```python
from build123d import *

# Parameters (mm, degrees)
F0_R      = 14.5
F1_DEPTH  = 25
F2_R      = 14.5
F3_DEPTH  = 3
F4_R      = 2.5
F5_DEPTH  = 25
F0_R_2    = 3
F6_DEPTH  = 30
F8_DEPTH  = 25
F9_DEPTH  = 3.5
F10_DEPTH = 30
F11_R     = 5


# Not quite as in the source:
# - a feature names something its author has since deleted; it is built from what else it names


with BuildPart() as f1:
    # F0 (on Top) → F1 (new body)
    with BuildSketch(Plane.XY):
        with BuildLine():
            Line((-44.2576195002, 24.5322410017), (-44.2576195002, -25.4677589983))
            Line((-44.2576195002, -25.4677589983), (-40.7576195002, -25.4677589983))
            Line((-40.7576195002, -25.4677589983), (-40.7576195002, 34.0321085225))
            Line((-40.7576195002, 34.0321085225), (26.7423804998, 34.0321085225))
            Line((26.7423804998, 34.0321085225), (26.7423804998, 19.5322410017))
            ThreePointArc((26.7423804998, 19.5322410017), (57.445862821, 6.7799260387), (44.8114401571, 37.5321085225))
            Line((44.8114401571, 37.5321085225), (44.6733208426, 37.5321085225))
            Line((44.6733208426, 37.5321085225), (-44.2576195002, 37.5321085225))
            Line((-44.2576195002, 37.5321085225), (-44.2576195002, 24.5322410017))
        make_face()
        with Locations((44.7423804998, 19.5322410017)):
            Circle(F0_R, mode=Mode.SUBTRACT)
    extrude(amount=F1_DEPTH)

    # F2 (on face) → F3 (join)
    with BuildSketch(Plane.XY.offset(25)):
        with BuildLine():
            ThreePointArc((26.7423804998, 19.5322410017), (29.5038185973, 9.9517279079), (36.9408506267, 3.3107696863))
            ThreePointArc((36.9408506267, 3.3107696863), (62.2844095115, 15.4977375434), (44.8114401571, 37.5321085225))
            Line((44.8114401571, 37.5321085225), (-44.2576195002, 37.5321085225))
            Line((-44.2576195002, 37.5321085225), (-44.2576195002, -25.4677589983))
            Line((-44.2576195002, -25.4677589983), (-40.7576195002, -25.4677589983))
            Line((-40.7576195002, -25.4677589983), (-40.7576195002, -15.0916781276))
            Line((-40.7576195002, -15.0916781276), (-40.7576195002, 34.0321085225))
            Line((-40.7576195002, 34.0321085225), (26.7423804998, 34.0321085225))
            Line((26.7423804998, 34.0321085225), (26.7423804998, 19.5322410017))
        make_face()
        with Locations((44.7423804998, 19.5322410017)):
            Circle(F2_R, mode=Mode.SUBTRACT)
    extrude(amount=-F3_DEPTH)

    # F4 (on face) → F5 (cut)
    with BuildSketch(Plane(origin=(-44.2576195002, 0, 0), x_dir=(0, -1, 0), z_dir=(-1, 0, 0))):
        with Locations((12.9677589983, 12.5)):
            Circle(F4_R)
    extrude(amount=-F5_DEPTH, mode=Mode.SUBTRACT)

    # F0 (on Top) → F6 (cut)
    with BuildSketch(Plane.XY):
        with Locations((44.7423804998, 19.5322410017)):
            Circle(F0_R_2)
    extrude(amount=F6_DEPTH, mode=Mode.SUBTRACT)

    # F4 (on face) → F8 (cut)
    with BuildSketch(Plane(origin=(-44.2576195002, 0, 0), x_dir=(0, -1, 0), z_dir=(-1, 0, 0))):
        with Locations((-22.0322410017, 12.5)):
            Circle(F4_R)
    extrude(amount=-F8_DEPTH, mode=Mode.SUBTRACT)

    # F2 (on face) → F9 (join)
    with BuildSketch(Plane.XY.offset(25)):
        with BuildLine():
            Line((18.9116307646, 10.5619383976), (36.9408506267, 3.3107696863))
            ThreePointArc((36.9408506267, 3.3107696863), (29.5038185973, 9.9517279079), (26.7423804998, 19.5322410017))
            Line((26.7423804998, 19.5322410017), (26.7423804998, 34.0321085225))
            Line((26.7423804998, 34.0321085225), (-40.7576195002, 34.0321085225))
            Line((-40.7576195002, 34.0321085225), (-40.7576195002, -15.0916781276))
            Line((-40.7576195002, -15.0916781276), (-14.5708816946, 10.5619383976))
            Line((-14.5708816946, 10.5619383976), (18.9116307646, 10.5619383976))
        make_face()
        with Locations((44.7423804998, 19.5322410017)):
            Circle(F2_R)
    extrude(amount=-F9_DEPTH)

    # F0 (on Top) → F10 (cut)
    with BuildSketch(Plane.XY):
        with Locations((44.7423804998, 19.5322410017)):
            Circle(F0_R_2)
    extrude(amount=F10_DEPTH, mode=Mode.SUBTRACT)

    # F11
    f11_edges = [f1.edges().sort_by_distance(p)[0] for p in [
        (26.74238, 34.032109, 10.75),
        (26.74238, 26.782175, 21.5),
        (-7.00762, 34.032109, 21.5),
        (-40.75762, 34.032109, 10.75),
        (-40.75762, 9.470215, 21.5),
    ]]
    fillet(f11_edges, radius=F11_R)


solid = f1.part
```
Source: CAD feature listing. Evaluate the final solid. Frame: model axes, mm. A direction names the side the tool comes from. Round coordinates to 2 decimals unless told otherwise and drop trailing zeros. Loops run counter-clockwise (first coordinate to the right, second up) from the corner with the lowest first, then second, coordinate; pieces in that order, holes last.
(1) Contact query for flat-ended pins moving along their axis: pin 1 Ø6 at (y, z) = (22.03, 12.5) entering from -X; pin 2 Ø1.5 at (x, z) = (-4.5, 12) entering from -Y; pin 3 Ø23 at (x, y) = (44.74, 19.53) entering from -Z; pin 4 Ø3 at (x, z) = (45, 12.5) entering from -Y. Output: stop coordinate, or through.
From the geometry:
pin 1: stops at x = -44.26
pin 2: stops at y = 34.03
pin 3: stops at z = 21.5
pin 4: stops at y = 1.53
(2) Material intervals for probe 1 along X at (y, z) = (13, 12.5); probe 2 along X at (y, z) = (21.5, 8); probe 3 along Y at (x, z) = (-31, 15.25), sorted ascending.
From the geometry:
probe 1: x = -44.26 to -40.76, 27.97 to 31.8, 57.69 to 61.52
probe 2: x = -44.26 to -40.76, 26.74 to 30.38, 59.11 to 62.63
probe 3: y = 34.03 to 37.53
(3) Section query D-D (y = -12.5). Output: boundary loops of the cut face in (x, z), and give its area (3 significant figures).
From the geometry:
outline: (-44.26, 0) - (-40.76, 0) - (-40.76, 10.04) - (-44.26, 10.04) - close; (-44.26, 14.96) - (-40.76, 14.96) - (-40.76, 16.5) arc R5 cw to (-38.11, 20.91) - (-38.11, 25) - (-44.26, 25) - close
area: 84.5 mm2
(4) Section query A-A (z = 12.5). Output: boundary loops of the cut face in (x, y).
From the geometry:
outline: (-44.26, -25.47) - (-40.76, -25.47) - (-40.76, -15.47) - (-44.26, -15.47) - close; (-44.26, -10.47) - (-40.76, -10.47) - (-40.76, 19.53) - (-44.26, 19.53) - close; (-44.26, 24.53) - (-40.76, 24.53) - (-40.76, 29.03) arc R5 cw to (-35.76, 34.03) - (21.74, 34.03) arc R5 cw to (26.74, 29.03) - (26.74, 19.53) arc R18 ccw (long way) to (44.81, 37.53) - (-44.26, 37.53) - close; hole circle Ø29 at (44.74, 19.53)
(5) Access query for faces 4 (the flat face through (48, 20, 21.5)), 5 (the flat face through (-7, 34.032, 8)), 6 (the flat face through (2, 10.562, 23)), 7 (the cylindrical face through (-42.53, 22.57, 10.06)). Directions: +Z, -Z, +X, -X, +Y, -Y. A direction counts if a zero-diameter tool reaches every point of the face in a straight line with its end or side. Return the directions, or none.
From the geometry:
face 4: -Z
face 5: -Z, -Y
face 6: +Z, -Z, -Y
face 7: -X
(6) Section query C-C (x = -10). Output: boundary loops of the cut face in (y, z).
From the geometry:
outline: (10.56, 21.5) - (29.03, 21.5) arc R5 cw to (34.03, 16.5) - (34.03, 0) - (37.53, 0) - (37.53, 25) - (10.56, 25) - close
(7) Section query B-B (z = 22.75). Output: boundary loops of the cut face in (x, y).
From the geometry:
outline: (-44.26, -25.47) - (-40.76, -25.47) - (-40.76, -15.09) - (-14.57, 10.56) - (18.91, 10.56) - (36.94, 3.31) arc R18 ccw (long way) to (44.81, 37.53) - (-44.26, 37.53) - close; hole circle Ø6 at (44.74, 19.53)
(8) Pull-direction query (Y, two-part tool) for faces 1 (the flat face through (8, 20, 25)), 2 (the flat face through (29.803, 6.181, 22.698)), 3 (the cylindrical face through (47.604, 20.433, 23.226)); classes: +Y half, -Y half, draft (parallel to the pull), parting line (faces both ways), or undercut.
From the geometry:
face 1: draft
face 2: -Y half
face 3: undercut
